For this review, use the dimensioned drawing (mm, ordinates from the lowest corner) and the shaded views. A direction names the side the tool comes from. Coordinates: 2 decimals unless noted, no trailing zeros. Write each loop counter-clockwise with the first axis right and the second up, starting at its lowest first coordinate (ties: lowest second). Pieces come first, ordered by that corner, then holes. Notation, with made-up numbers: (40, -31) - (85, -31) arc R31 cw to (85, 6) - close; hole circle Ø6 at (0.25, 46.25). An arc over 180 degrees is marked (long way). Answer as a JSON object with one key per item and string values.
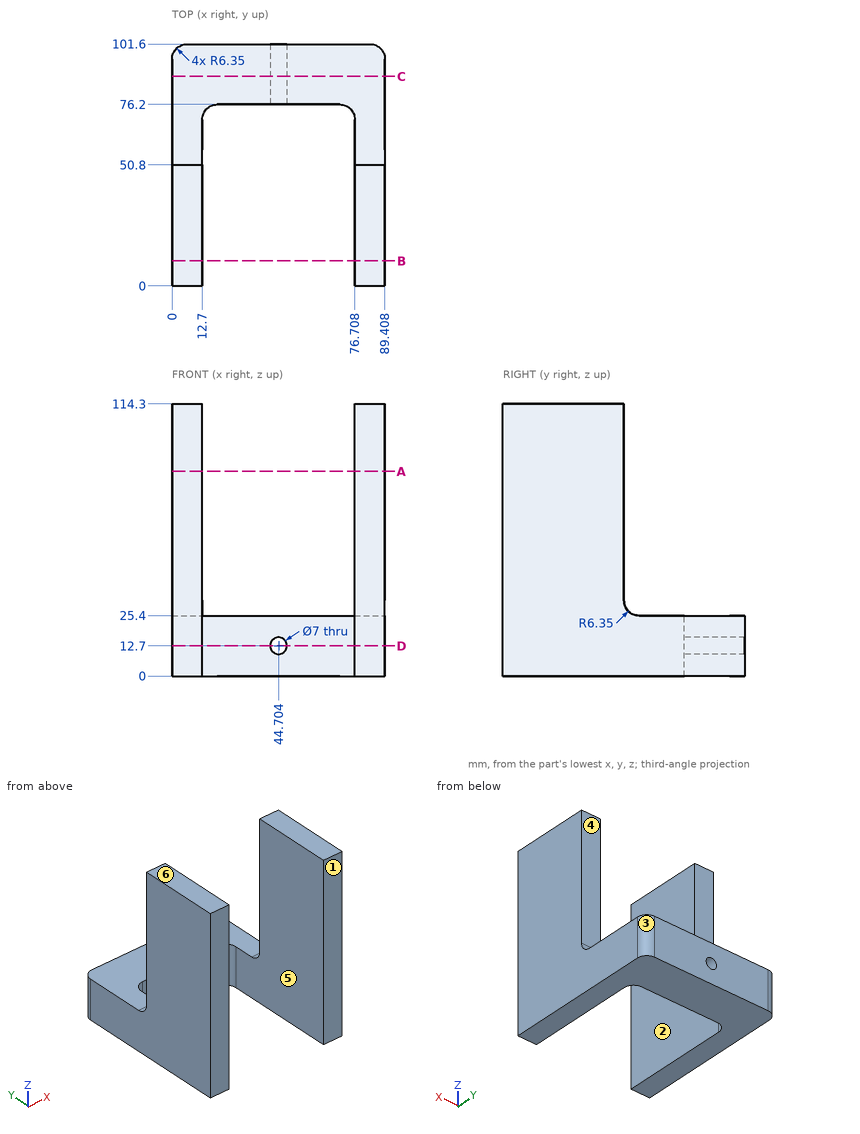
(1) Tool access review of the marked faces 4, 5 and 6: name each direction out of +Z, -Z, +X, -X, +Y, -Y from which nothing blocks a thin tool from reaching the whole face with its end or side.
Solved:
{"face 4": "+Z, +X, -X, +Y", "face 5": "+Z, -Z, -Y", "face 6": "+Z, +X, -X, +Y, -Y"}
(2) To check wall thickness, follow line 1 (X direction, y = 20, z = 81); line 2 (X direction, y = 94, z = 12.7); line 3 (Y direction, x = 83, z = 108). State the ranges of each line that lie inside material, in increasing order. Write a range as from..to.
Solved:
{"line 1": "x = 0..12.7, 76.71..89.41", "line 2": "x = 0..41.2, 48.2..89.41", "line 3": "y = 0..50.8"}
(3) Take a section at D-D, the plane z = 12.7. Write out the cut boundary in (x, y), and give its area (3 significant figures).
Solved:
{"outline": "(0, 0) - (12.7, 0) - (12.7, 69.85) arc R6.35 cw to (19.05, 76.2) - (41.2, 76.2) - (41.2, 101.6) - (6.35, 101.6) arc R6.35 ccw to (0, 95.25) - close; (48.2, 76.2) - (70.36, 76.2) arc R6.35 cw to (76.71, 69.85) - (76.71, 0) - (89.41, 0) - (89.41, 95.25) arc R6.35 ccw to (83.06, 101.6) - (48.2, 101.6) - close", "area": "4,030 mm^2"}
(4) Take a section at C-C, the plane y = 88. Write out the cut boundary in (x, z).
Solved:
{"outline": "(0, 0) - (89.41, 0) - (89.41, 25.4) - (0, 25.4) - close; hole circle Ø7 at (44.7, 12.7)"}
(5) For pin 1 (8 mm diameter, centred on x = 44.704, z = 12.7, fed in from -Y); pin 2 (4 mm diameter, centred on x = 6.5, z = 76.5, fed in from +Y); pin 3 (2 mm diameter, centred on x = 78, y = 78.5, fed in from -Z), all flat-tipped, find the tip position at first contact; note any pin that passes through.
Solved:
{"pin 1": "stops at y = 76.2", "pin 2": "stops at y = 50.8", "pin 3": "stops at z = 0"}
(6) The part is to be moulded in two halves that separate along X. For the marked faces 1, 2 and 3, say which applies: pulls with the +X half, pulls with the -X half, needs draft (parallel to the pull), parting line crosses it, or undercut.
Solved:
{"face 1": "needs draft", "face 2": "undercut", "face 3": "pulls with the +X half"}
(7) Take a section at A-A, the plane z = 86. Write out the cut boundary in (x, y).
Solved:
{"outline": "(0, 0) - (12.7, 0) - (12.7, 50.8) - (0, 50.8) - close; (76.71, 0) - (89.41, 0) - (89.41, 50.8) - (76.71, 50.8) - close"}
(8) Take a section at B-B, the plane y = 10.5. Write out the cut boundary in (x, z).
Solved:
{"outline": "(0, 0) - (12.7, 0) - (12.7, 114.3) - (0, 114.3) - close; (76.71, 0) - (89.41, 0) - (89.41, 114.3) - (76.71, 114.3) - close"}
